from build123d import *

# Parameters (mm, degrees)
SKETCH_1_W          = 50
SKETCH_1_H          = 45.4
SKETCH_1_R          = 1.6
EXTRUDE_1_DEPTH     = 4
SKETCH_2_W          = 12
SKETCH_2_H          = 0.4
EXTRUDE_2_DEPTH     = 45.4
CHAMFER_1_SIZE      = 0.4
SKETCH_3_W          = 50
SKETCH_3_H          = 9
CUT_EXTRUDE_1_DEPTH = 0.4
SKETCH_4_R          = 1.6
CUT_EXTRUDE_2_DEPTH = 68.654711588
SKETCH_5_W          = 8.6
SKETCH_5_H          = 15
EXTRUDE_3_DEPTH     = 4
SKETCH_6_R          = 1.6
CUT_EXTRUDE_3_DEPTH = 4


with BuildPart() as part:
    # 草图1 → 凸台-拉伸1 (new body)
    with BuildSketch(Plane(origin=(0, 0, 0), x_dir=(1, 0, 0), z_dir=(0, 1, 0))):
        with Locations((25, 22.7)):
            Rectangle(SKETCH_1_W, SKETCH_1_H)
        with Locations(Location((15, 32.7, 0), (0, 0, 270))):
            Circle(SKETCH_1_R, mode=Mode.SUBTRACT)
        with Locations(Location((35, 32.7, 0), (0, 0, 270))):
            Circle(SKETCH_1_R, mode=Mode.SUBTRACT)
        with Locations(Location((35, 12.7, 0), (0, 0, 270))):
            Circle(SKETCH_1_R, mode=Mode.SUBTRACT)
        with Locations(Location((15, 12.7, 0), (0, 0, 270))):
            Circle(SKETCH_1_R, mode=Mode.SUBTRACT)
    extrude(amount=EXTRUDE_1_DEPTH)

    # 草图2 → 凸台-拉伸2 (add)
    with BuildSketch(Plane.XY):
        with Locations((25, 4.2)):
            Rectangle(SKETCH_2_W, SKETCH_2_H)
    extrude(amount=-EXTRUDE_2_DEPTH)

    # 倒角1
    chamfer_1_edges = [part.edges().sort_by_distance(p)[0] for p in [
        (31, 4, -22.7),
        (19, 4, -22.7),
    ]]
    chamfer(chamfer_1_edges, length=CHAMFER_1_SIZE - 0.0001)  # a hair under: the kernel refuses the full size

    # 草图3 → 切除-拉伸1 (cut)
    with BuildSketch(Plane(origin=(0, 0, 0), x_dir=(-1, 0, 0), z_dir=(0, -1, 0))):
        with Locations((-25, 22.7)):
            Rectangle(SKETCH_3_W, SKETCH_3_H)
    extrude(amount=-CUT_EXTRUDE_1_DEPTH, mode=Mode.SUBTRACT)

    # 草图4 → 切除-拉伸2 (cut, through all)
    with BuildSketch(Plane(origin=(0, 0.4, 0), x_dir=(-1, 0, 0), z_dir=(0, -1, 0))):
        with Locations(Location((-5, 22.7, 0), (0, 0, 90))):
            Circle(SKETCH_4_R)
        with Locations(Location((-25, 22.7, 0), (0, 0, 90))):
            Circle(SKETCH_4_R)
        with Locations(Location((-45, 22.7, 0), (0, 0, 90))):
            Circle(SKETCH_4_R)
    extrude(amount=-CUT_EXTRUDE_2_DEPTH, mode=Mode.SUBTRACT)

    # 草图5 → 凸台-拉伸3 (add)
    with BuildSketch(Plane(origin=(0, 4, 0), x_dir=(1, 0, 0), z_dir=(0, 1, 0))):
        with Locations((45.7, 52.9)):
            Rectangle(SKETCH_5_W, SKETCH_5_H)
    extrude(amount=-EXTRUDE_3_DEPTH)

    # 草图6 → 切除-拉伸3 (cut)
    with BuildSketch(Plane.XZ):
        with Locations(Location((45.7, -56.9, 0), (0, 0, 270))):
            Circle(SKETCH_6_R)
        with Locations(Location((45.7, -36.1, 0), (0, 0, 270))):
            Circle(SKETCH_6_R)
    extrude(amount=-CUT_EXTRUDE_3_DEPTH, mode=Mode.SUBTRACT)


solid = part.part
Part model, mm, in its own coordinate system. A direction names the side the tool comes from. Give positions to 0.01 mm unless a question says otherwise; leave off trailing zeros. Order: outer loops, then holes, each group sorted by start corner. A loop starts at its lowest first (then second) coordinate and runs counter-clockwise, first axis right, second up. Notation, with made-up numbers: (-36, 76.5) - (2, 76.5) arc R33 ccw to (2, 114.5) - close; hole circle Ø8 at (-34.75, 42). An arc over 180 degrees is marked (long way). Use a Markdown table: item, result.
1) Two-plate mould, pull along X, no slides. Class faces 1 (the flat face through (50, 2, -30)), 2 (the cylindrical face through (15.481, 1.972, -31.174)), 3 (the flat face through (41.4, 2, -53)), 4 (the flat face through (41, 4, -24)): +X half, -X half, draft (parallel to the pull), parting line (faces both ways), or undercut.
Checked values:
| item | result |
|---|---|
| face 1 | +X half |
| face 2 | undercut |
| face 3 | -X half |
| face 4 | draft |
2) Saw through at C-C on x = 5. List the corners of the cut face in (y, z).
Checked values:
| item | result |
|---|---|
| outline | (0, -45.4) - (4, -45.4) - (4, -24.3) - (0.4, -24.3) - (0.4, -27.2) - (0, -27.2) - close; (0, -18.2) - (0.4, -18.2) - (0.4, -21.1) - (4, -21.1) - (4, 0) - (0, 0) - close |
3) 3-axis set-ups, long thin cutter, end or side, ignore diameter. For faces 5 (the flat face through (9, 4, -23)), 6 (the flat face through (25.3, 0.4, -20.8)), 7 (the cylindrical face through (25.481, 2.372, -24.226)): which of +Z, -Z, +X, -X, +Y, -Y reach the whole face in a straight line?
Checked values:
| item | result |
|---|---|
| face 5 | +Z, -Z, -X, +Y |
| face 6 | +X, -X, -Y |
| face 7 | +Y, -Y |
4) Flat gauge pins, fed straight in: P1, Ø2.5, axis at x = 35, z = -12.7, coming from the +Y side; P2, Ø4, axis at x = 5, z = -22.7, coming from the +Y side; P3, Ø4, axis at x = 45, z = -22.7, coming from the -Y side; P4, Ø1, axis at x = 27.5, y = 0.5, coming from the -Z side. Where does each tip first touch, or does it go through?
Checked values:
| item | result |
|---|---|
| P1 | through |
| P2 | y = 4 |
| P3 | y = 0.4 |
| P4 | z = -45.4 |
5) Saw through at B-B on z = -22.7. Count the separate pieces of the cut face and the enclosed holes in it, plus the area to 3 significant figures.
Checked values:
| item | result |
|---|---|
| separate pieces | 4 |
| enclosed holes | 0 |
| area | 149 mm² |
6) Probe L1, parallel to X at y = 1.4, z = -22.7; L2, parallel to X at y = 1.2, z = -32.7; L3, parallel to Z at x = 14.5, y = 2. List the from-to ranges inside material, lowest first. Write a range as from..to.
Checked values:
| item | result |
|---|---|
| L1 | 0..3.4, 6.6..23.4, 26.6..43.4, 46.6..50 |
| L2 | 0..13.4, 16.6..33.4, 36.6..50 |
| L3 | -45.4..-34.22, -31.18..-14.22, -11.18..0 |
7) Saw through at A-A on z = -56.9. List the corners of the cut face in (x, y), plus the area to 3 significant figures.
Checked values:
| item | result |
|---|---|
| outline | (41.4, 0) - (44.1, 0) - (44.1, 4) - (41.4, 4) - close; (47.3, 0) - (50, 0) - (50, 4) - (47.3, 4) - close |
| area | 21.6 mm² |
